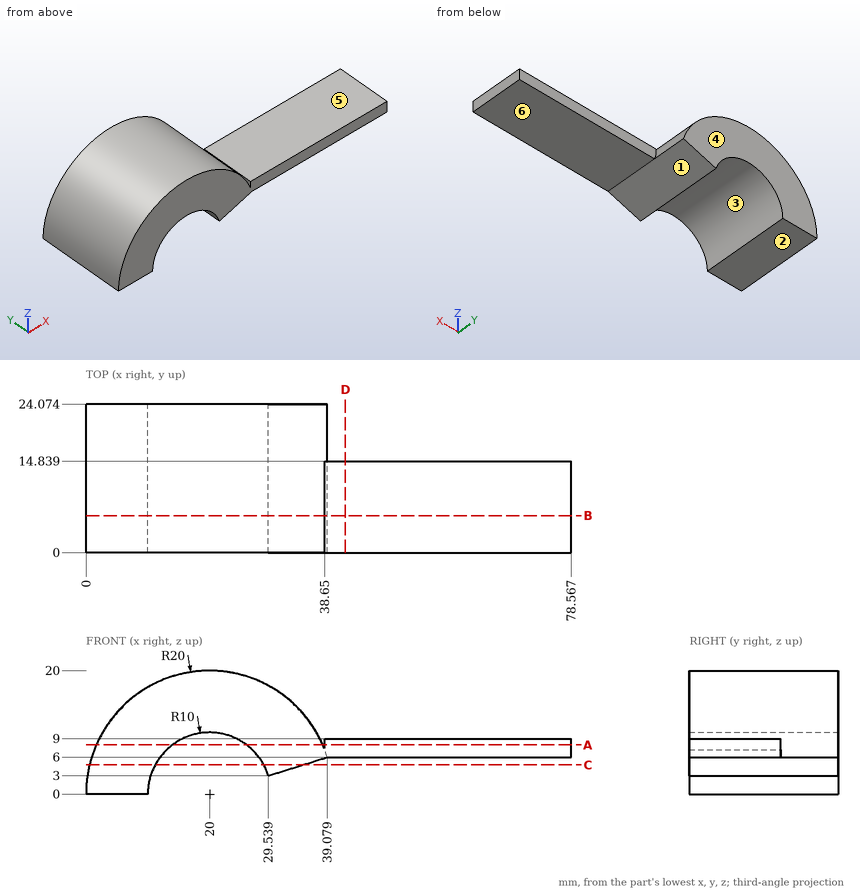
Part print with two shaded views. Sizes in mm from the minimum x, y, z corner. A direction names the side the tool comes from. Coordinates: 2 decimals unless noted, no trailing zeros. Write each loop counter-clockwise with the first axis right and the second up, starting at its lowest first coordinate (ties: lowest second). Pieces come first, ordered by that corner, then holes. Notation, with made-up numbers: (73, 34) -> (89, 34) arc R27 cw to (89, 52) -> close; hole circle Ø3 at (-13.75, 76). An arc over 180 degrees is marked (long way). Return JSON: item names as keys, results as strings. Group by question number.
Q1. Drill centre lines: line 1 (Z direction, x = 48, y = 6.5); line 2 (X direction, y = 2, z = 6.5) (1 decimal); line 3 (X direction, y = 10.75, z = 1.5). Where is each one in solid material? Low to high.
Q2. Cut at D-D, the plane x = 42. Give the cut face in (y, z).
Q3. Which spindle directions (+Z, -Z, +X, -X, +Y, -Y) get a long thin tool onto all of the face, cutting with end or side? Do the marked faces 4, 5 and 6. Say none if no direction does.
Q4. Cut at A-A, the plane z = 8. State how many separate pieces and enclosed holes the cut face has, then the cut area to 3 significant figures.
Q5. Pull direction X, two halves, no side cores. Call the marked faces 1, 2 and 3: released by +X, released by -X, zero draft, split by the parting line, or undercut.
Q6. Cut at C-C, the plane z = 4.75. Give the cut face in (x, y) (1 decimal).
Q7. Cut at B-B, the plane y = 6. Give the cut face in (x, z), then the cut area to 3 significant figures.
Q8. Flat gauge pins, fed straight in: pin 1 (0.5 mm diameter, centred on y = 7.5, z = 8.5, fed in from -X); pin 2 (1 mm diameter, centred on x = 69, y = 12, fed in from +Z); pin 3 (1.5 mm diameter, centred on x = 68.5, z = 7, fed in from +Y). Where does each tip first touch, or does it go through?
Returned:
{
 "1": {"line 1": "z = 6 to 9", "line 2": "x = 1.1 to 12.4, 27.6 to 78.6", "line 3": "x = 0.06 to 10.11"},
 "2": {"outline": "(0, 6) -> (14.84, 6) -> (14.84, 9) -> (0, 9) -> close"},
 "3": {"face 4": "+Z, -Z, +X, -X, +Y", "face 5": "+Z, +X, +Y, -Y", "face 6": "-Z, +X, +Y, -Y"},
 "4": {"separate pieces": "3", "enclosed holes": "0", "area": "1,190 mm2"},
 "5": {"face 1": "released by +X", "face 2": "zero draft", "face 3": "undercut"},
 "6": {"outline": "(0.6, 0) -> (11.2, 0) -> (11.2, 24.1) -> (0.6, 24.1) -> close; (28.8, 0) -> (35.1, 0) -> (35.1, 24.1) -> (28.8, 24.1) -> close"},
 "7": {"outline": "(0, 0) -> (10, 0) arc R10 cw to (29.54, 3) -> (39.08, 6) -> (78.57, 6) -> (78.57, 9) -> (38.65, 9) -> (38.65, 7.22) arc R20 ccw to start", "area": "545 mm2"},
 "8": {"pin 1": "stops at x = 1.78", "pin 2": "stops at z = 9", "pin 3": "stops at y = 14.84"}
}
